Design review of the part shown in the three views and the two pictorial views. Dimensions are in mm from the part's minimum x, y and z. Give positions to 0.01 mm unless a question says otherwise; leave off trailing zeros. Loops run counter-clockwise (first coordinate to the right, second up) from the corner with the lowest first, then second, coordinate; pieces in that order, holes last.
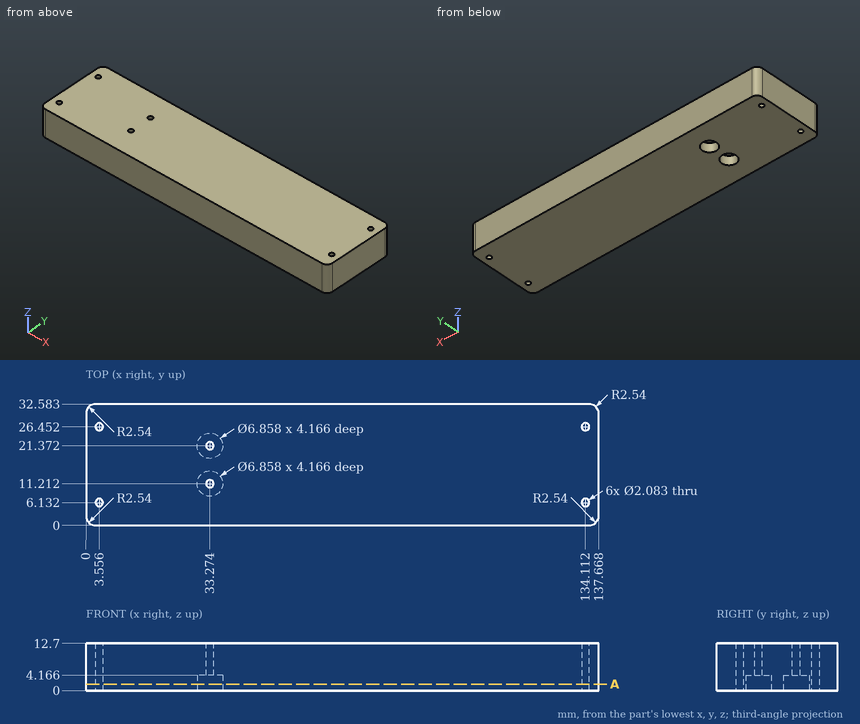
Q1. Consider section A-A on z = 1.75. Give the boundary of the cut face in (x, y).
Answers:
outline: (0, 2.54) arc R2.54 ccw to (2.54, 0) - (135.13, 0) arc R2.54 ccw to (137.67, 2.54) - (137.67, 30.04) arc R2.54 ccw to (135.13, 32.58) - (2.54, 32.58) arc R2.54 ccw to (0, 30.04) - close; hole circle Ø2.08 at (3.56, 6.13); hole circle Ø2.08 at (3.56, 26.45); hole circle Ø6.86 at (33.27, 11.21); hole circle Ø6.86 at (33.27, 21.37); hole circle Ø2.08 at (134.11, 6.13); hole circle Ø2.08 at (134.11, 26.45)
Q2. For probe 1 along Y at (x, z) = (31.5, 3) (1 decimal); probe 2 along X at (y, z) = (11, 3.75); probe 3 along X at (y, z) = (6.5, 3.25) (1 decimal), list the stretches that pass through material, from the lowest coordinate up.
Answers:
probe 1: y = 0 to 8.3, 14.1 to 18.4, 24.3 to 32.6
probe 2: x = 0 to 29.85, 36.7 to 137.67
probe 3: x = 0 to 2.6, 4.5 to 133.1, 135.1 to 137.7
Q3. For pin 1 Ø2 at (x, y) = (33, 21) entering from -Z, flat-tipped, find the tip position at first contact; note if it passes through.
Answers:
pin 1: stops at z = 4.17
